from build123d import *

# Parameters (mm, degrees)
DIA_CYLINDRE_R = 7.5
CYLINDRE_DEPTH = 33.5
CHANFREIN_SIZE = 0.5


with BuildPart() as part:
    # Dia cylindre → Cylindre (new body, symmetric)
    with BuildSketch(Plane.XY):
        Circle(DIA_CYLINDRE_R)
    extrude(amount=CYLINDRE_DEPTH, both=True)

    # Chanfrein
    chanfrein_edges = [part.edges().sort_by_distance(p)[0] for p in [
        (-7.5, 0, -33.5),
        (-7.5, 0, 33.5),
    ]]
    chamfer(chanfrein_edges, length=CHANFREIN_SIZE)

    # Profil rainure → Rainure (revolve, cut)
    with BuildSketch(Plane(origin=(0, 0, 0), x_dir=(1, 0, 0), z_dir=(0, 1, 0))):
        Polygon((-7.5, 1.5), (-7.5, -1.5), (-6, 0), align=None)
    revolve(axis=Axis((0, 0, -36.430134701), (0, 0, 1)), mode=Mode.SUBTRACT)


solid = part.part
Input: part model. Units: mm. Frame: model coordinates. Coordinates: 2 decimals unless noted, no trailing zeros. Loops run counter-clockwise (first coordinate to the right, second up) from the corner with the lowest first, then second, coordinate; pieces in that order, holes last.
(1) Section A-A on z = 27.5. Return the cut outline in (x, y), then the cut area to 3 significant figures.
(2) First-contact query: pin 1 Ø1.5 at (y, z) = (4, -5.5) entering from +X; pin 2 Ø3 at (x, z) = (-1.5, -10.5) entering from -Y; pin 3 Ø3 at (y, z) = (5.5, -6) entering from +X; pin 4 Ø1.5 at (x, z) = (-1.5, 19.5) entering from +Y. Flat tips, straight axial feed; report the tip coordinate or a pass-through.
(3) Material intervals for probe 1 along Z at (x, y) = (-3.5, 5.25); probe 2 along X at (y, z) = (-5.5, 2); probe 3 along X at (y, z) = (-2, -9.5), sorted ascending.
Data:
1. outline: circle Ø15 at (0, 0)
1. area: 177 mm2
2. pin 1: stops at x = 6.76
2. pin 2: stops at y = -7.5
2. pin 3: stops at x = 6.34
2. pin 4: stops at y = 7.46
3. probe 1: z = -33.5 to -0.31, 0.31 to 33.5
3. probe 2: x = -5.1 to 5.1
3. probe 3: x = -7.23 to 7.23
